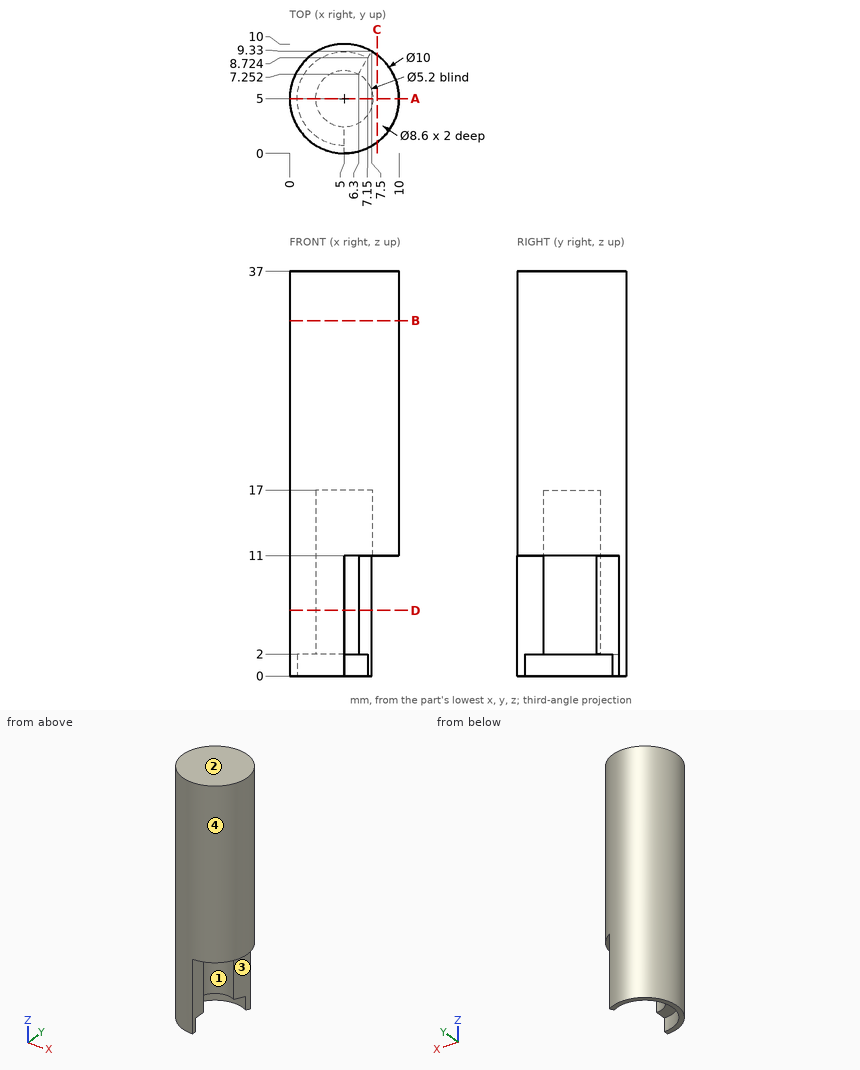
The figure shows three views and two pictorial views of one solid part (mm, origin at its lowest corner). Answer the questions. Give positions to 0.01 mm unless a question says otherwise; leave off trailing zeros. Write each loop counter-clockwise with the first axis right and the second up, starting at its lowest first coordinate (ties: lowest second). Pieces come first, ordered by that corner, then holes. Notation, with made-up numbers: M 67.25,80 L 126.25,80 A17 cw 126.25,103 Z; hole C 66.25,37.5 d2. An arc over 180 degrees is marked long. One line per item, written item: value. Start each with the question number.
(1) Find section A-A (y = 5). Determine the outline of the cut face in (x, z).
(2) Find section C-C (x = 8). Determine the outline of the cut face in (y, z).
(3) Find section D-D (z = 6). Determine the outline of the cut face in (x, y).
(4) Determine the mould class of the marked faces 1, 2, 3 and 4 for opening direction Y: pulls with the +Y half, pulls with the -Y half, needs draft (parallel to the pull), parting line crosses it, or undercut.
(5) Find section B-B (z = 32.5). Determine the outline of the cut face in (x, y).
(6) Flat-ended cylindrical pins translate along their axes: pin 1 Ø1.5 at (x, y) = (4.5, 4) entering from -Z; pin 2 Ø1.5 at (y, z) = (2.5, 9) entering from -X; pin 3 Ø5.5 at (x, y) = (7.5, 3) entering from -Z. Find the tip coordinate at first contact, or state that the pin passes through.
(7) Find the intervals of material crossed by line 1 (Z direction, x = 7.25, y = 5.75); line 2 (Z direction, x = 5, y = 8); line 3 (X direction, y = 5, z = 1.4), in increasing order.
Results below:
1. outline: M 0,0 L 0.7,0 L 0.7,2 L 2.4,2 L 2.4,17 L 7.6,17 L 7.6,11 L 10,11 L 10,37 L 0,37 Z
2. outline: M 1,11 L 9,11 L 9,37 L 1,37 Z
3. outline: M 5,0 L 5,2.4 A2.6 cw long 6.3,7.25 L 7.5,9.33 A5 ccw long Z
4. face 1: undercut
4. face 2: needs draft
4. face 3: pulls with the -Y half
4. face 4: parting line crosses it
5. outline: C 5,5 d10
6. pin 1: stops at z = 17
6. pin 2: stops at x = 0.32
6. pin 3: stops at z = 2
7. line 1: z = 17 to 37
7. line 2: z = 2 to 37
7. line 3: x = 0 to 0.7
